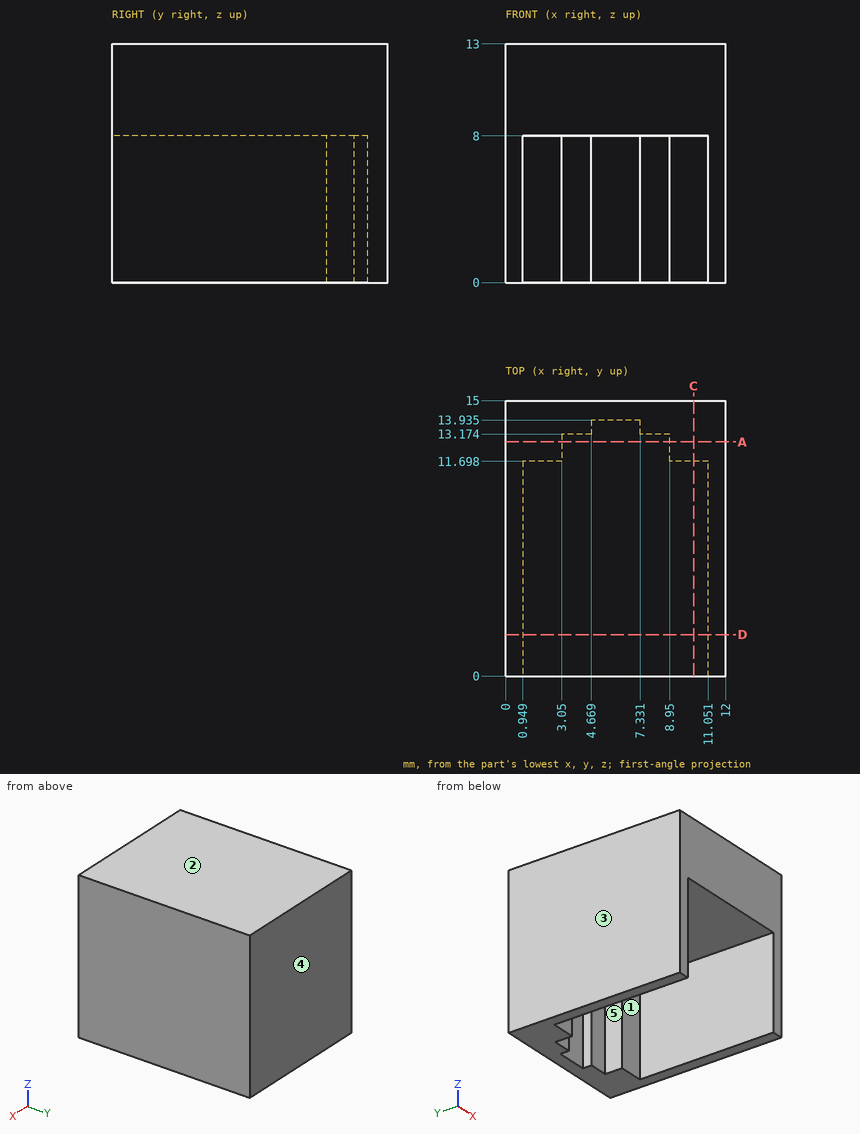
Geometry check sheet. Reference: drawing and pictorial views, mm from the part's lowest x, y, z. A direction names the side the tool comes from. Give positions to 0.01 mm unless a question says otherwise; leave off trailing zeros. Loops run counter-clockwise (first coordinate to the right, second up) from the corner with the lowest first, then second, coordinate; pieces in that order, holes last. Notation, with made-up numbers: (80.5, 33.25) - (135.5, 33.25) arc R27 ccw to (135.5, 70.25) - close; hole circle Ø11 at (22, 38). An arc over 180 degrees is marked (long way). Use CSV: the item, a comma, the result in double quotes. Start each with the question number.
Q1. Section check C-C, the plane x = 10.25. Record the cut outline in (y, z).
Q2. Scan lines: probe 1 along X at (y, z) = (6.75, 1); probe 2 along X at (y, z) = (13.75, 4.5); probe 3 along Y at (x, z) = (5, 6) (1 decimal). Record each from-to range of solid material in increasing order. Write a range as from..to.
Q3. Release check for a two-part mould opening along X. For the marked faces 3, 4 and 5 record: +X half, -X half, draft (parallel to the pull), parting line (faces both ways), or undercut.
Q4. Access from +Z, -Z, +X, -X, +Y, -Y to the whole of each face (thin tool, end or side, straight path). Record for the marked faces 1 and 2.
Q5. Section check D-D, the plane y = 2.25. Record the cut outline in (x, z).
Q6. Section check A-A, the plane y = 12.75. Record the cut outline in (x, z), and give its area (3 significant figures).
Q7. Go/stop test with flat-tipped pins: pin 1 Ø1.5 at (x, z) = (9.5, 6) entering from -Y; pin 2 Ø0.6 at (y, z) = (13.5, 5) entering from -X; pin 3 Ø3 at (x, z) = (5.5, 2.5) entering from -Y; pin 4 Ø3 at (x, y) = (6.5, 7) entering from -Z. Record where each tip stops, or that it passes through.
Findings below:
1,outline,"(0, 8) - (11.7, 8) - (11.7, 0) - (15, 0) - (15, 13) - (0, 13) - close"
2,probe 1,"x = 0..0.95, 11.05..12"
2,probe 2,"x = 0..4.67, 7.33..12"
2,probe 3,"y = 13.9..15"
3,face 3,"-X half"
3,face 4,"draft"
3,face 5,"undercut"
4,face 1,"-Z, -Y"
4,face 2,"+Z, +X, -X, +Y, -Y"
5,outline,"(0, 0) - (0.95, 0) - (0.95, 8) - (11.05, 8) - (11.05, 0) - (12, 0) - (12, 13) - (0, 13) - close"
6,outline,"(0, 0) - (3.05, 0) - (3.05, 8) - (8.95, 8) - (8.95, 0) - (12, 0) - (12, 13) - (0, 13) - close"
6,area,"109 mm^2"
7,pin 1,"stops at y = 11.7"
7,pin 2,"stops at x = 0"
7,pin 3,"stops at y = 13.17"
7,pin 4,"stops at z = 8"
